from build123d import *

# Parameters (mm, degrees)
F0_W     = 6.5
F0_H     = 24
F0_R     = 1.475
F1_DEPTH = 3


with BuildPart() as f1:
    # F0 (on Right) → F1 (new body)
    with BuildSketch(Plane.YZ):
        Rectangle(F0_W, F0_H)
        with Locations((0, -3.5)):
            Circle(F0_R, mode=Mode.SUBTRACT)
        with Locations((0, 6.9)):
            Circle(F0_R, mode=Mode.SUBTRACT)
    extrude(amount=F1_DEPTH)


solid = f1.part
Build history of the part. All positions in model axes, mm. Coordinates: 2 decimals unless noted, no trailing zeros. Write each loop counter-clockwise with the first axis right and the second up, starting at its lowest first coordinate (ties: lowest second). Pieces come first, ordered by that corner, then holes.
(1) Mould opens along Y. For faces 1 (the flat face through (1, 3.25, 0)), 2 (the cylindrical face through (1.48, -0.32, 5.46)), 3 (the flat face through (3, 0, 0)), 4 (the flat face through (1, -3.25, 0)) say: pulls with the +Y half, pulls with the -Y half, needs draft (parallel to the pull), parting line crosses it, or undercut.
(2) Cut at B-B on z = 6.9. List the corners of the cut face in (x, y) (3 decimals), and give its area (4 significant figures).
(3) Drill centre lines: line 1 (Z direction, x = 2.2, y = 0) (3 decimals); line 2 (Z direction, x = 1.6, y = -0.5); line 3 (Y direction, x = 1.4, z = -2.5). Where is each one in solid material? Low to high.
(4) Cut at C-C on x = 1.25. List the corners of the cut face in (y, z) (3 decimals), and give its area (3 significant figures).
(5) Cut at A-A on y = 0. List the corners of the cut face in (x, z) (3 decimals), and give its area (3 significant figures).
(6) Pin check, flat tip, straight feed: pin 1 Ø3 at (y, z) = (-0.5, -9) entering from -X. Stop position of the tip, or through.
Working result:
1. face 1: pulls with the +Y half
1. face 2: undercut
1. face 3: needs draft
1. face 4: pulls with the -Y half
2. outline: (0, -3.25) - (3, -3.25) - (3, -1.475) - (0, -1.475) - close; (0, 1.475) - (3, 1.475) - (3, 3.25) - (0, 3.25) - close
2. area: 10.65 mm2
3. line 1: z = -12 to -4.975, -2.025 to 5.425, 8.375 to 12
3. line 2: z = -12 to -4.89, -2.11 to 5.51, 8.29 to 12
3. line 3: y = -3.25 to -1.08, 1.08 to 3.25
4. outline: (-3.25, -12) - (3.25, -12) - (3.25, 12) - (-3.25, 12) - close; hole circle Ø2.95 at (0, -3.5); hole circle Ø2.95 at (0, 6.9)
4. area: 142 mm2
5. outline: (0, -12) - (3, -12) - (3, -4.975) - (0, -4.975) - close; (0, -2.025) - (3, -2.025) - (3, 5.425) - (0, 5.425) - close; (0, 8.375) - (3, 8.375) - (3, 12) - (0, 12) - close
5. area: 54.3 mm2
6. pin 1: stops at x = 0
